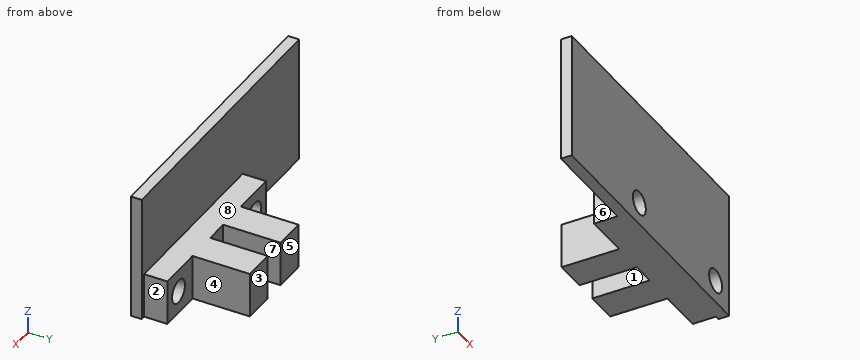
from build123d import *

# Parameters (mm, degrees)
SKETCH1_W           = 39
SKETCH1_H           = 17.4
BOSS_EXTRUDE1_DEPTH = 1.5
SKETCH2_W           = 24.4
SKETCH2_H           = 6.2
BOSS_EXTRUDE2_DEPTH = 3.2
SKETCH3_W           = 4.4
SKETCH3_H           = 6.2
BOSS_EXTRUDE3_DEPTH = 7.9
SKETCH4_R           = 1.6
CUT_EXTRUDE1_DEPTH  = 23.767301114


with BuildPart() as part:
    # Sketch1 → Boss-Extrude1 (new body)
    with BuildSketch(Plane(origin=(0, 0, 0), x_dir=(1, 0, 0), z_dir=(0, 1, 0))):
        Rectangle(SKETCH1_W, SKETCH1_H)
    extrude(amount=BOSS_EXTRUDE1_DEPTH)

    # Sketch2 → Boss-Extrude2 (add)
    with BuildSketch(Plane(origin=(0, 1.5, 0), x_dir=(1, 0, 0), z_dir=(0, 1, 0))):
        with Locations((6.7, 5.6)):
            Rectangle(SKETCH2_W, SKETCH2_H)
    extrude(amount=BOSS_EXTRUDE2_DEPTH)

    # Sketch3 → Boss-Extrude3 (add)
    with BuildSketch(Plane(origin=(0, 4.7, 0), x_dir=(1, 0, 0), z_dir=(0, 1, 0))):
        with Locations((2.9, 5.6)):
            Rectangle(SKETCH3_W, SKETCH3_H)
        with Locations((10.5, 5.6)):
            Rectangle(SKETCH3_W, SKETCH3_H)
    extrude(amount=BOSS_EXTRUDE3_DEPTH)

    # Sketch4 → Cut-Extrude1 (cut, through all)
    with BuildSketch(Plane(origin=(0, 4.7, 0), x_dir=(1, 0, 0), z_dir=(0, 1, 0))):
        with Locations(Location((-2.75, 5.6, 0), (0, 0, 270))):
            Circle(SKETCH4_R)
        with Locations(Location((16.15, 5.6, 0), (0, 0, 270))):
            Circle(SKETCH4_R)
    extrude(amount=-CUT_EXTRUDE1_DEPTH, mode=Mode.SUBTRACT)


solid = part.part
Can you work these out from the model? Positions are in its coordinate system, mm. Face numbers are marked on the shaded views. A direction names the side the tool comes from. Give positions to 0.01 mm unless a question says otherwise; leave off trailing zeros. Loops run counter-clockwise (first coordinate to the right, second up) from the corner with the lowest first, then second, coordinate; pieces in that order, holes last. Notation, with made-up numbers: (68, -14.75) -> (76, -14.75) arc R21 cw to (76, -3.75) -> close; hole circle Ø9 at (84.25, 68.25). An arc over 180 degrees is marked (long way). Return JSON: item names as keys, results as strings.
Q1. On a 3-axis mill with a long thin cutter (end or side, diameter ignored), from which of +Z, -Z, +X, -X, +Y, -Y can I reach the whole of each face in a straight line? I mean the marked faces 4, 5, 6, 7 and 8. Say none if no direction works.
Checks:
{"face 4": "+Z, -Z, +X, +Y", "face 5": "+Z, -Z, +X, -X, +Y", "face 6": "+Z, -Z, -X, +Y", "face 7": "+Z, -Z, +Y", "face 8": "+Z, +X, -X, +Y"}
Q2. I want a section at B-B, the plane x = -2.75. List the corners of the cut face in (y, z) for me.
Checks:
{"outline": "(0, -8.7) -> (4.7, -8.7) -> (4.7, -7.2) -> (0, -7.2) -> close; (0, -4) -> (4.7, -4) -> (4.7, -2.5) -> (1.5, -2.5) -> (1.5, 8.7) -> (0, 8.7) -> close"}
Q3. I want a section at C-C, the plane y = 5.75. List the corners of the cut face in (x, z) for me, then the cut area to 3 significant figures.
Checks:
{"outline": "(0.7, -8.7) -> (5.1, -8.7) -> (5.1, -2.5) -> (0.7, -2.5) -> close; (8.3, -8.7) -> (12.7, -8.7) -> (12.7, -2.5) -> (8.3, -2.5) -> close", "area": "54.6 mm2"}
Q4. I need wall thicknesses on probe 1 along X at (y, z) = (2.7, -5.6); probe 2 along X at (y, z) = (1.1, -5.6); probe 3 along X at (y, z) = (7.75, -4). Which ranges of each line are inside material? Lowest first, please.
Checks:
{"probe 1": "x = -5.5 to -4.35, -1.15 to 14.55, 17.75 to 18.9", "probe 2": "x = -19.5 to -4.35, -1.15 to 14.55, 17.75 to 19.5", "probe 3": "x = 0.7 to 5.1, 8.3 to 12.7"}
Q5. For pin 1 Ø1.9 at (x, z) = (-3, -6.5) entering from +Y; pin 2 Ø1.6 at (y, z) = (3, -6) entering from -X; pin 3 Ø2 at (x, z) = (5.5, 4.5) entering from +Y; pin 4 Ø3 at (x, z) = (-2.75, -5.6) entering from +Y, each with a flat end and sliding along its axis, tell me the tip position at first contact or that it passes through.
Checks:
{"pin 1": "stops at y = 4.7", "pin 2": "stops at x = -5.5", "pin 3": "stops at y = 1.5", "pin 4": "passes through"}
Q6. I want a section at D-D, the plane y = 2.75. List the corners of the cut face in (x, z) for me.
Checks:
{"outline": "(-5.5, -8.7) -> (18.9, -8.7) -> (18.9, -2.5) -> (-5.5, -2.5) -> close; hole circle Ø3.2 at (-2.75, -5.6); hole circle Ø3.2 at (16.15, -5.6)"}
Q7. I want a section at A-A, the plane z = -5.6. List the corners of the cut face in (x, y) for me.
Checks:
{"outline": "(-19.5, 0) -> (-4.35, 0) -> (-4.35, 4.7) -> (-5.5, 4.7) -> (-5.5, 1.5) -> (-19.5, 1.5) -> close; (-1.15, 0) -> (14.55, 0) -> (14.55, 4.7) -> (12.7, 4.7) -> (12.7, 12.6) -> (8.3, 12.6) -> (8.3, 4.7) -> (5.1, 4.7) -> (5.1, 12.6) -> (0.7, 12.6) -> (0.7, 4.7) -> (-1.15, 4.7) -> close; (17.75, 0) -> (19.5, 0) -> (19.5, 1.5) -> (18.9, 1.5) -> (18.9, 4.7) -> (17.75, 4.7) -> close"}
Q8. We'd pull the mould along X, two halves only. Please class the marked faces 1, 2 and 3: released by +X, released by -X, zero draft, split by the parting line, or undercut.
Checks:
{"face 1": "undercut", "face 2": "released by +X", "face 3": "zero draft"}
